Input: part model. Units: mm. Frame: model coordinates. A direction names the side the tool comes from. Coordinates: 2 decimals unless noted, no trailing zeros. Order: outer loops, then holes, each group sorted by start corner. A loop starts at its lowest first (then second) coordinate and runs counter-clockwise, first axis right, second up. Notation, with made-up numbers: M -27,88.5 L -13,88.5 A17 ccw -13,103.5 Z; hole C 73,18.5 d2. An arc over 180 degrees is marked long. One line per item, written item: value.
```python
from build123d import *

# Parameters (mm, degrees)
F0_W     = 215.9
F0_H     = 139.7
F1_DEPTH = 5.08


with BuildPart() as f1:
    # F0 (on Top) → F1 (new body)
    with BuildSketch(Plane.XY):
        with Locations((-51.475366, 25.492683)):
            Rectangle(F0_W, F0_H)
        Polygon((-111.475366, -34.507317), (-111.475366, 25.492683), (-111.475366, 85.492683), (-51.475366, 85.492683), (8.524634, 85.492683), (8.524634, 25.492683), (8.524634, -34.507317), (-51.475366, -34.507317), align=None, mode=Mode.SUBTRACT)
    extrude(amount=F1_DEPTH)


solid = f1.part
```
(1) Cut plane B-B on z = 1.95. Output: boundary loops of the cut face in (x, y), plus the area to 3 significant figures.
Data:
outline: M -159.43,-44.36 L 56.47,-44.36 L 56.47,95.34 L -159.43,95.34 Z; hole M -111.48,-34.51 L 8.52,-34.51 L 8.52,85.49 L -111.48,85.49 Z
area: 15,800 mm2
(2) Cut plane A-A on y = 73.5. Output: boundary loops of the cut face in (x, z).
Data:
outline: M -159.43,0 L -111.48,0 L -111.48,5.08 L -159.43,5.08 Z; M 8.52,0 L 56.47,0 L 56.47,5.08 L 8.52,5.08 Z
(3) Access query for faces 4 (the flat face through (-51, -34.507, 3)), 5 (the flat face through (-53, -36, 0)). Directions: +Z, -Z, +X, -X, +Y, -Y. A direction counts if a zero-diameter tool reaches every point of the face in a straight line with its end or side. Return the directions, or none.
Data:
face 4: +Z, -Z
face 5: -Z, +X, -X, +Y, -Y
(4) Draft query along Y for faces 1 (the flat face through (-159.425, 25, 3)), 2 (the flat face through (8.525, 26, 3)), 3 (the flat face through (-53, 95.343, 3)). Return one class per face: released by +Y, released by -Y, zero draft, split by the parting line, or undercut.
Data:
face 1: zero draft
face 2: undercut
face 3: released by +Y
(5) Cut plane C-C on x = -7. Output: boundary loops of the cut face in (y, z), plus the area to 3 significant figures.
Data:
outline: M -44.36,0 L -34.51,0 L -34.51,5.08 L -44.36,5.08 Z; M 85.49,0 L 95.34,0 L 95.34,5.08 L 85.49,5.08 Z
area: 100 mm2
(6) Ray query, line 1 (X direction, y = 11.5, z = 2.65); line 2 (Y direction, x = -50, z = 1.2). Return the intervals inside material, ascending. Write a range as from..to.
Data:
line 1: x = -159.43..-111.48, 8.52..56.47
line 2: y = -44.36..-34.51, 85.49..95.34
